Here's how the part is built. I have some questions about the finished solid (model axes, mm). A direction names the side the tool comes from. Round coordinates to 2 decimals unless told otherwise and drop trailing zeros. Order: outer loops, then holes, each group sorted by start corner. A loop starts at its lowest first (then second) coordinate and runs counter-clockwise, first axis right, second up. Notation, with made-up numbers: M 25,8.5 L 41,8.5 A27 ccw 41,27.5 Z; hole C -29,-12.5 d1. An arc over 180 degrees is marked long. Write item = value, one per line. Start each with the question number.
Item 1: I'm going to push flat-ended pins straight in: P1, Ø10, axis at x = 2, y = 9.5, coming from the +Z side; P2, Ø2.5, axis at x = 6, y = 28, coming from the -Z side. Where does each tip first touch, or does it pass through?
Item 2: Please list where these lines run through material, in increasing order: L1, parallel to Y at x = -8, z = 1.25; L2, parallel to Y at x = 36, z = 5.
Item 3: I want a section at A-A, the plane z = 6.5. List the corners of the cut face in (x, y) for me, plus the area to 3 significant figures.
Item 4: We'd pull the mould along X, two halves only. Please class faces 4 (the face through (-1, -38, 0)), 5 (the face through (-45.14, -45.1, 4.56)), 6 (the face through (-42, -1, 7)): pulls with the +X half, pulls with the -X half, needs draft (parallel to the pull), parting line crosses it, or undercut.
Item 5: I want a section at C-C, the plane x = -34.5. List the corners of the cut face in (y, z) for me.
Item 6: For faces 1 (the face through (-1, 46, 4)), 2 (the face through (-1, 27, 2)), 3 (the face through (42, -1, 7)), which set-ups out of +Z, -Z, +X, -X, +Y, -Y let a thin tool reach every point of the face, with its end or its side?
Item 7: I want a section at B-B, the plane y = 32. List the corners of the cut face in (x, z) for me, plus the area to 3 significant figures.
```python
from build123d import *

# Parameters (mm, degrees)
SKETCH_W        = 92
SKETCH_H        = 92
PAD_DEPTH       = 9
SKETCH001_W     = 84
SKETCH001_H     = 84
POCKET_DEPTH    = 5
FILLET_R        = 3
SKETCH002_W     = 92
SKETCH002_H     = 5
POCKET001_DEPTH = 2


with BuildPart() as part:
    # Sketch → Pad (new body)
    with BuildSketch(Plane.XY):
        Rectangle(SKETCH_W, SKETCH_H)
    extrude(amount=PAD_DEPTH)

    # Sketch001 (on Face6 of Pad) → Pocket (cut)
    with BuildSketch(Plane.XY.offset(9)):
        Rectangle(SKETCH001_W, SKETCH001_H)
    extrude(amount=-POCKET_DEPTH, mode=Mode.SUBTRACT)

    # Fillet
    fillet_edges = [part.edges().sort_by_distance(p)[0] for p in [
        (-46, 46, 4.5),
        (-46, -46, 4.5),
        (46, -46, 4.5),
        (46, 46, 4.5),
    ]]
    fillet(fillet_edges, radius=FILLET_R)

    # Sketch002 (on Face2 of Fillet) → Pocket001 (cut)
    with BuildSketch(Plane(origin=(0, 0, 0), x_dir=(1, 0, 0), z_dir=(0, 0, -1))):
        with Locations((0, 27.5)):
            Rectangle(SKETCH002_W, SKETCH002_H)
        with Locations((0, -27.5)):
            Rectangle(SKETCH002_W, SKETCH002_H)
    extrude(amount=-POCKET001_DEPTH, mode=Mode.SUBTRACT)


solid = part.part
```
Filled in:
q1.P1 = 4
q1.P2 = 2
q2.L1 = -46 to -30, -25 to 25, 30 to 46
q2.L2 = -46 to -42, 42 to 46
q3.outline = M -46,-43 A3 ccw -43,-46 L 43,-46 A3 ccw 46,-43 L 46,43 A3 ccw 43,46 L -43,46 A3 ccw -46,43 Z; hole M -42,-42 L 42,-42 L 42,42 L -42,42 Z
q3.area = 1,400 mm^2
q4.face_4 = needs draft
q4.face_5 = pulls with the -X half
q4.face_6 = undercut
q5.outline = M -46,0 L -30,0 L -30,2 L -25,2 L -25,0 L 25,0 L 25,2 L 30,2 L 30,0 L 46,0 L 46,9 L 42,9 L 42,4 L -42,4 L -42,9 L -46,9 Z
q6.face_1 = +Z, -Z, +X, -X, +Y
q6.face_2 = -Z, +X, -X
q6.face_3 = +Z
q7.outline = M -46,0 L 46,0 L 46,9 L 42,9 L 42,4 L -42,4 L -42,9 L -46,9 Z
q7.area = 408 mm^2
